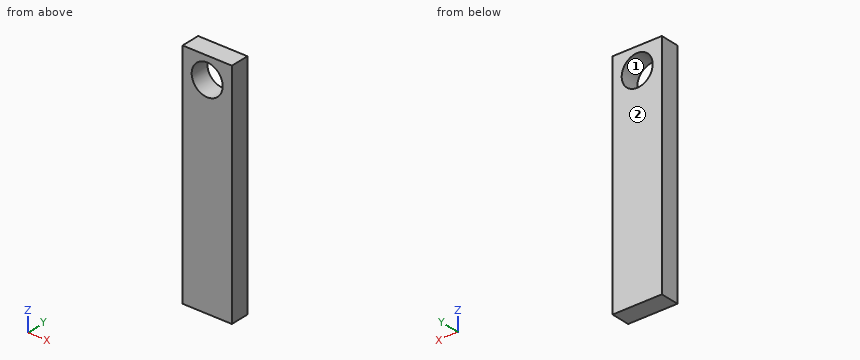
```python
from build123d import *

# Parameters (mm, degrees)
SKETCH1_R           = 2.07899
BOSS_EXTRUDE1_DEPTH = 2.54


with BuildPart() as part:
    # Sketch1 → Boss-Extrude1 (new body)
    with BuildSketch(Plane(origin=(0, 0, 0), x_dir=(1, 0, 0), z_dir=(0, 1, 0))):
        Polygon((0, 0), (6.618, 0), (6.618, -25.450703704), (6.618, -30.796997366), (0, -30.796997366), (0, -27.9), (0, -25.450703704), align=None)
        with Locations((3.309, -27.9)):
            Circle(SKETCH1_R, mode=Mode.SUBTRACT)
    extrude(amount=BOSS_EXTRUDE1_DEPTH)


solid = part.part
```
The model under review builds one solid part; all positions refer to its coordinate system, in mm. Face numbers are marked on the shaded views. Coordinates: 2 decimals unless noted, no trailing zeros. Write each loop counter-clockwise with the first axis right and the second up, starting at its lowest first coordinate (ties: lowest second). Pieces come first, ordered by that corner, then holes. Notation, with made-up numbers: (14.5, 6) - (67.5, 6) arc R24 cw to (67.5, 45) - close; hole circle Ø1 at (51.25, 22.5). An arc over 180 degrees is marked (long way). Answer in a Markdown table with one row per item. Add a question column.
Q1. Consider section A-A on z = 27.9. Give the boundary of the cut face in (x, y).
Q2. To check wall thickness, follow line 1 along X through (y, z) = (1.1, 27.9); line 2 along Z through (x, y) = (4.5, 1.85); line 3 along Z through (x, y) = (4, 1). State the ranges of each line that lie inside material, in increasing order. Write a range as from..to.
Q3. Consider section B-B on x = 3.5. Give the boundary of the cut face in (y, z).
Q4. Clearance check with a flat-ended pin moving along its axis: pin 1 (3.5 mm diameter, centred on x = 3.309, z = 27.9, fed in from -Y) (1 decimal). State where the tip first meets the part, or that it passes through.
Q5. Draft analysis for pull direction X (two halves, no side actions). For the marked faces 1 and 2, state which applies: +X half, -X half, draft (parallel to the pull), parting line (faces both ways), or undercut.
Q6. Consider section C-C on y = 1.3. Give the boundary of the cut face in (x, z), then the cut area to 3 significant figures.
Answers below:
| question | item | result |
|---|---|---|
| 1 | outline | (0, 0) - (1.23, 0) - (1.23, 2.54) - (0, 2.54) - close; (5.39, 0) - (6.62, 0) - (6.62, 2.54) - (5.39, 2.54) - close |
| 2 | line 1 | 0..1.23, 5.39..6.62 |
| 2 | line 2 | 0..26.2, 29.6..30.8 |
| 2 | line 3 | 0..25.94, 29.86..30.8 |
| 3 | outline | (0, 0) - (2.54, 0) - (2.54, 25.83) - (0, 25.83) - close; (0, 29.97) - (2.54, 29.97) - (2.54, 30.8) - (0, 30.8) - close |
| 4 | pin 1 | through |
| 5 | face 1 | undercut |
| 5 | face 2 | draft |
| 6 | outline | (0, 0) - (6.62, 0) - (6.62, 30.8) - (0, 30.8) - close; hole circle Ø4.16 at (3.31, 27.9) |
| 6 | area | 190 mm² |
